from build123d import *

# Parameters (mm, degrees)
F1_DEPTH = 100
F2_R     = 0.5


with BuildPart() as f1:
    # F0 (on Top) → F1 (new body)
    with BuildSketch(Plane.XY):
        Polygon((-36.73992, 8.346775), (-38.73992, 8.346775), (-38.73992, -6.87493), (-11.73992, -6.87493), (-11.73992, 8.346775), (-13.73992, 8.346775), (-14.23992, -3.87493), (-16.23992, -3.87493), (-16.73992, 8.346775), (-18.73992, 8.346775), (-19.23992, -3.87493), (-21.23992, -3.87493), (-21.73992, 8.346775), (-23.73992, 8.346775), (-24.23992, -3.87493), (-26.23992, -3.87493), (-26.73992, 8.346775), (-28.73992, 8.346775), (-29.23992, -3.87493), (-31.23992, -3.87493), (-31.73992, 8.346775), (-33.73992, 8.346775), (-34.23992, -3.87493), (-36.23992, -3.87493), align=None)
    extrude(amount=F1_DEPTH)

    # F2
    f2_edges = [f1.edges().sort_by_distance(p)[0] for p in [
        (-13.73992, 8.346775, 50),
        (-11.73992, 8.346775, 50),
        (-18.73992, 8.346775, 50),
        (-16.73992, 8.346775, 50),
        (-23.73992, 8.346775, 50),
        (-21.73992, 8.346775, 50),
        (-28.73992, 8.346775, 50),
        (-26.73992, 8.346775, 50),
        (-33.73992, 8.346775, 50),
        (-31.73992, 8.346775, 50),
        (-38.73992, 8.346775, 50),
        (-36.73992, 8.346775, 50),
        (-36.23992, -3.87493, 50),
        (-33.98992, 2.235922, 100),
        (-31.23992, -3.87493, 50),
        (-26.23992, -3.87493, 50),
        (-24.23992, -3.87493, 50),
        (-29.23992, -3.87493, 50),
        (-21.23992, -3.87493, 50),
        (-19.23992, -3.87493, 50),
        (-16.23992, -3.87493, 50),
        (-14.23992, -3.87493, 50),
    ]]
    fillet(f2_edges, radius=F2_R)


solid = f1.part
Verification items for the finished model (mm, model axes). A direction names the side the tool comes from. Coordinates: 2 decimals unless noted, no trailing zeros. One line per item, written item: value. Start each with the question number.
Item 1: Access from +Z, -Z, +X, -X, +Y, -Y to the whole of each face (thin tool, end or side, straight path). Record for faces 1 (the flat face through (-38.74, 1, 49)), 2 (the flat face through (-24, 2, 49)).
Item 2: Scan lines: probe 1 along X at (y, z) = (4.5, 12.5); probe 2 along X at (y, z) = (-2, 62.5); probe 3 along Y at (x, z) = (-20.5, 66.5). Record each from-to range of solid material in increasing order.
Item 3: Mould release check, pull along X, two halves, no side actions. Record for faces 3 (the flat face through (-11.74, 0, 49)), 4 (the flat face through (-22, -1, 0)), 5 (the flat face through (-34, 2, 49)): released by +X, released by -X, zero draft, split by the parting line, or undercut.
Item 4: Sectioned sample at A-A (y = 3.75). Count the separate pieces of the cut face and the enclosed holes in it, then the cut area to 3 significant figures.
Item 5: Gauge pin test, flat ends, axial feed: pin 1 (0.5 mm diameter, centred on x = -30.5, z = 65, fed in from +Y); pin 2 (5 mm diameter, centred on x = -18.5, y = -4, fed in from -Z). Record the tip position at first contact, or that the pin passes through.
Conclusion:
1. face 1: +Z, -Z, -X, +Y, -Y
1. face 2: +Z, -Z, +Y
2. probe 1: x = -38.74 to -36.58, -33.9 to -31.58, -28.9 to -26.58, -23.9 to -21.58, -18.9 to -16.58, -13.9 to -11.74
2. probe 2: x = -38.74 to -36.32, -34.16 to -31.32, -29.16 to -26.32, -24.16 to -21.32, -19.16 to -16.32, -14.16 to -11.74
2. probe 3: y = -6.87 to -3.87
3. face 3: released by +X
3. face 4: zero draft
3. face 5: undercut
4. separate pieces: 6
4. enclosed holes: 0
4. area: 1,390 mm^2
5. pin 1: stops at y = -3.87
5. pin 2: stops at z = 0
